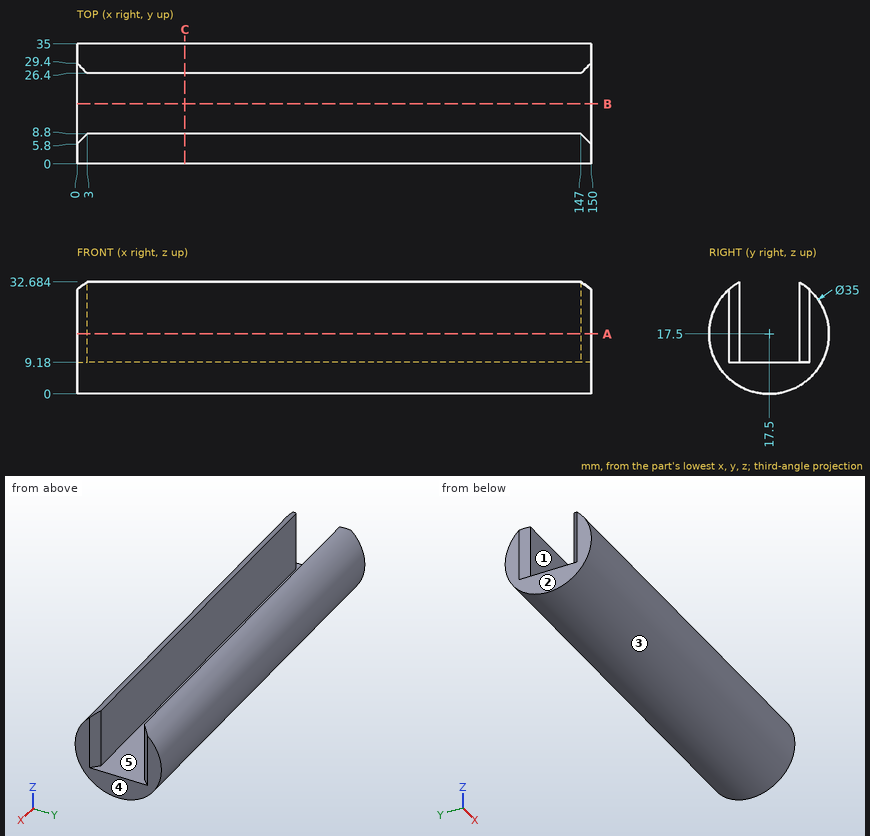
Drawing for the job (mm, zero at the part's lowest x, y, z). A direction names the side the tool comes from. Round coordinates to 2 decimals unless told otherwise and drop trailing zeros. Loops run counter-clockwise (first coordinate to the right, second up) from the corner with the lowest first, then second, coordinate; pieces in that order, holes last.
1. Band-saw the part on B-B, the plane y = 17.5. List the corners of the cut face in (x, z), and give its area (3 significant figures).
Check values:
outline: (0, 0) - (150, 0) - (150, 9.18) - (0, 9.18) - close
area: 1,380 mm2
2. Mould opens along Y. For the marked faces 3, 4 and 5 say: +Y half, -Y half, draft (parallel to the pull), parting line (faces both ways), or undercut.
Check values:
face 3: parting line
face 4: draft
face 5: undercut
3. Band-saw the part on C-C, the plane x = 31.5. List the corners of the cut face in (y, z).
Check values:
outline: (8.8, 9.18) - (8.8, 32.68) arc R17.5 ccw (long way) to (26.4, 32.57) - (26.4, 9.18) - close
4. Drop flat-ended pins along their axis: P1, Ø1, axis at x = 64.5, z = 4, coming from the -Y side (1 decimal); P2, Ø8, axis at x = 46.5, z = 8, coming from the +Y side; P3, Ø12, axis at x = 50.5, z = 6, coming from the -Y side. Give the stop position or say it passes through.
Check values:
P1: stops at y = 5.8
P2: stops at y = 34.11
P3: stops at y = 0.89
5. Tool access for the marked faces 1 and 2: list every direction of +Z, -Z, +X, -X, +Y, -Y with a clear straight run to the whole face (end or side of a thin tool).
Check values:
face 1: +Z, +X, -X
face 2: +Z, -Z, -X, +Y, -Y
6. Band-saw the part on A-A, the plane z = 17.5. List the corners of the cut face in (x, y).
Check values:
outline: (0, 0) - (150, 0) - (150, 5.8) - (147, 8.8) - (3, 8.8) - (0, 5.8) - close; (0, 29.4) - (3, 26.4) - (147, 26.4) - (150, 29.4) - (150, 35) - (0, 35) - close
7. Wall check: probe 1 along Y at (x, z) = (86, 23); probe 2 along Y at (x, z) = (71, 17); probe 3 along Z at (x, y) = (108.5, 18). Give the ranges that are in metal, low to high.
Check values:
probe 1: y = 0.89 to 8.8, 26.4 to 34.11
probe 2: y = 0.01 to 8.8, 26.4 to 34.99
probe 3: z = 0.01 to 9.18
